The model under review builds one solid part; all positions refer to its coordinate system, in mm. A direction names the side the tool comes from. Give positions to 0.01 mm unless a question says otherwise; leave off trailing zeros. Order: outer loops, then holes, each group sorted by start corner. A loop starts at its lowest first (then second) coordinate and runs counter-clockwise, first axis right, second up.
```python
from build123d import *

# Parameters (mm, degrees)
SKETCH1_W                                       = 45
SKETCH1_H                                       = 50
BOSS_EXTRUDE1_DEPTH                             = 16
CUT_EXTRUDE1_DEPTH                              = 58.116109812
SKETCH4_W                                       = 24
SKETCH4_H                                       = 50
CUT_EXTRUDE2_DEPTH                              = 0.72
CUT_EXTRUDE3_DEPTH                              = 58.116109812
SKETCH8_R                                       = 7.5
CUT_EXTRUDE4_DEPTH                              = 0.72
CSK_FOR_M6_FLAT_HEAD_MACHINE_SCREW1_D           = 7
CSK_FOR_M6_FLAT_HEAD_MACHINE_SCREW1_CSINK_D     = 12.6
CSK_FOR_M6_FLAT_HEAD_MACHINE_SCREW1_CSINK_ANGLE = 90
CUT_EXTRUDE5_DEPTH                              = 2.5
FILLET1_R                                       = 1
FILLET2_R                                       = 1
FILLET4_R                                       = 0.5
CUT_EXTRUDE7_DEPTH                              = 11.5
SKETCH18_R                                      = 2.75
CUT_EXTRUDE8_DEPTH                              = 14.5
SKETCH19_R                                      = 2.75
CUT_EXTRUDE9_DEPTH                              = 10
SKETCH21_W                                      = 8.99
SKETCH21_H                                      = 50
BOSS_EXTRUDE2_DEPTH                             = 0.6
CHAMFER1_SIZE                                   = 4
FILLET5_R                                       = 1
CHAMFER2_SIZE                                   = 1


with BuildPart() as part:
    # Sketch1 → Boss-Extrude1 (new body)
    with BuildSketch(Plane(origin=(0, 0, 0), x_dir=(1, 0, 0), z_dir=(0, 1, 0))):
        Rectangle(SKETCH1_W, SKETCH1_H)
    extrude(amount=BOSS_EXTRUDE1_DEPTH)

    # Sketch3 → Cut-Extrude1 (cut, through all)
    with BuildSketch(Plane.XY.offset(25)):
        Polygon((-13.5, 16), (-17.5, 12), (22.5, 12), (22.5, 16), align=None)
    extrude(amount=-CUT_EXTRUDE1_DEPTH, mode=Mode.SUBTRACT)

    # Sketch4 → Cut-Extrude2 (cut)
    with BuildSketch(Plane(origin=(0, 12, 0), x_dir=(1, 0, 0), z_dir=(0, 1, 0))):
        with Locations((2.5, 0)):
            Rectangle(SKETCH4_W, SKETCH4_H)
    extrude(amount=-CUT_EXTRUDE2_DEPTH, mode=Mode.SUBTRACT)

    # Sketch5 → Cut-Extrude3 (cut, through all)
    with BuildSketch(Plane.XY.offset(25)):
        Polygon((-22.5, 16), (-13.5, 16), (-13.51, 15.99), (-22.5, 15.99), align=None)
    extrude(amount=-CUT_EXTRUDE3_DEPTH, mode=Mode.SUBTRACT)

    # Sketch8 → Cut-Extrude4 (cut)
    with BuildSketch(Plane(origin=(0, 11.28, 0), x_dir=(1, 0, 0), z_dir=(0, 1, 0))):
        with Locations(Location((2.5, 0, 0), (0, 0, 180))):
            Circle(SKETCH8_R)
    extrude(amount=-CUT_EXTRUDE4_DEPTH, mode=Mode.SUBTRACT)

    # CSK for M6 Flat Head Machine Screw1 (through all)
    with Locations(Plane(origin=(0, 10.56, 0), x_dir=(1, 0, 0), z_dir=(0, 1, 0))):
        with Locations((2.5, 0)):
            CounterSinkHole(CSK_FOR_M6_FLAT_HEAD_MACHINE_SCREW1_D / 2, CSK_FOR_M6_FLAT_HEAD_MACHINE_SCREW1_CSINK_D / 2, counter_sink_angle=CSK_FOR_M6_FLAT_HEAD_MACHINE_SCREW1_CSINK_ANGLE)

    # Sketch12 → Cut-Extrude5 (cut)
    with BuildSketch(Plane(origin=(0, 11.28, 0), x_dir=(1, 0, 0), z_dir=(0, 1, 0))):
        with BuildLine():
            Line((7.5, 16.6), (-2.5, 16.6))
            ThreePointArc((-2.5, 16.6), (-3.207106781, 16.892893219), (-3.5, 17.6))
            Line((-3.5, 17.6), (-3.5, 25))
            Line((-3.5, 25), (8.5, 25))
            Line((8.5, 25), (8.5, 17.6))
            ThreePointArc((8.5, 17.6), (8.207106781, 16.892893219), (7.5, 16.6))
        make_face()
    cut_extrude5 = extrude(amount=-CUT_EXTRUDE5_DEPTH, mode=Mode.SUBTRACT)

    # Fillet1
    fillet1_edges = [part.edges().sort_by_distance(p)[0] for p in [
        (-3.5, 10.03, -25),
        (8.5, 10.03, -25),
    ]]
    fillet(fillet1_edges, radius=FILLET1_R)

    # Mirror2: Cut-Extrude5 across plane
    add(cut_extrude5.mirror(Plane.XY), mode=Mode.SUBTRACT)

    # Fillet2
    # the kernel refuses this fillet: 1 mm, written as the material it takes off along each edge
    with BuildSketch(Plane(origin=(7.5, 11.28, 17.6), x_dir=(1, 0, 0), z_dir=(0, 0, 1))) as fillet2_piece_1:
        with BuildLine():
            CenterArc((1 + FILLET2_R, -FILLET2_R), FILLET2_R, 90, 90)
            Line((1, -FILLET2_R), (1 - FILLET2_R * 0.02, -FILLET2_R))
            Line((1 - FILLET2_R * 0.02, -FILLET2_R), (1 - FILLET2_R * 0.02, FILLET2_R * 0.02))
            Line((1 - FILLET2_R * 0.02, FILLET2_R * 0.02), (1 + FILLET2_R, FILLET2_R * 0.02))
            Line((1 + FILLET2_R, FILLET2_R * 0.02), (1 + FILLET2_R, 0))
        make_face()
    revolve(axis=Axis((7.5, 11.28, 17.6), (0, 1, 0)), revolution_arc=90, mode=Mode.SUBTRACT)
    with BuildSketch(Plane(origin=(8.5, 11.28, 27.5), x_dir=(1, 0, 0), z_dir=(0, 0, -1)), Plane(origin=(-3.5, 11.28, 17.6), x_dir=(-1, 0, 0), z_dir=(0, 0, 1))) as fillet2_piece_2:
        with BuildLine():
            CenterArc((FILLET2_R, FILLET2_R), FILLET2_R, 180, 90)
            Line((0, FILLET2_R), (-FILLET2_R * 0.02, FILLET2_R))
            Line((-FILLET2_R * 0.02, FILLET2_R), (-FILLET2_R * 0.02, -FILLET2_R * 0.02))
            Line((-FILLET2_R * 0.02, -FILLET2_R * 0.02), (FILLET2_R, -FILLET2_R * 0.02))
            Line((FILLET2_R, -FILLET2_R * 0.02), (FILLET2_R, 0))
        make_face()
    extrude(amount=9.9, mode=Mode.SUBTRACT)
    with BuildSketch(Plane(origin=(-2.5, 11.28, 17.6), x_dir=(0, 0, -1), z_dir=(1, 0, 0))) as fillet2_piece_3:
        with BuildLine():
            CenterArc((1 + FILLET2_R, -FILLET2_R), FILLET2_R, 90, 90)
            Line((1, -FILLET2_R), (1 - FILLET2_R * 0.02, -FILLET2_R))
            Line((1 - FILLET2_R * 0.02, -FILLET2_R), (1 - FILLET2_R * 0.02, FILLET2_R * 0.02))
            Line((1 - FILLET2_R * 0.02, FILLET2_R * 0.02), (1 + FILLET2_R, FILLET2_R * 0.02))
            Line((1 + FILLET2_R, FILLET2_R * 0.02), (1 + FILLET2_R, 0))
        make_face()
    revolve(axis=Axis((-2.5, 11.28, 17.6), (0, 1, 0)), revolution_arc=90, mode=Mode.SUBTRACT)
    with BuildSketch(Plane(origin=(7.5, 11.28, 16.6), x_dir=(0, 0, -1), z_dir=(-1, 0, 0))) as fillet2_piece_4:
        with BuildLine():
            CenterArc((FILLET2_R, FILLET2_R), FILLET2_R, 180, 90)
            Line((0, FILLET2_R), (-FILLET2_R * 0.02, FILLET2_R))
            Line((-FILLET2_R * 0.02, FILLET2_R), (-FILLET2_R * 0.02, -FILLET2_R * 0.02))
            Line((-FILLET2_R * 0.02, -FILLET2_R * 0.02), (FILLET2_R, -FILLET2_R * 0.02))
            Line((FILLET2_R, -FILLET2_R * 0.02), (FILLET2_R, 0))
        make_face()
    extrude(amount=10, mode=Mode.SUBTRACT)
    with BuildSketch(Plane(origin=(-4.5, 11.28, -25), x_dir=(0, 0, 1), z_dir=(-1, 0, 0)), Plane(origin=(14.5, 11.28, -25), x_dir=(0, 0, 1), z_dir=(-1, 0, 0))) as fillet2_piece_5:
        with BuildLine():
            CenterArc((FILLET2_R, -FILLET2_R), FILLET2_R, 90, 90)
            Line((0, -FILLET2_R), (-FILLET2_R * 0.02, -FILLET2_R))
            Line((-FILLET2_R * 0.02, -FILLET2_R), (-FILLET2_R * 0.02, FILLET2_R * 0.02))
            Line((-FILLET2_R * 0.02, FILLET2_R * 0.02), (FILLET2_R, FILLET2_R * 0.02))
            Line((FILLET2_R, FILLET2_R * 0.02), (FILLET2_R, 0))
        make_face()
    extrude(amount=5, mode=Mode.SUBTRACT)
    with BuildSketch(Plane(origin=(2.5, 11.28, 0), x_dir=(-1, 0, 0), z_dir=(0, 0, -1))) as fillet2_piece_6:
        with BuildLine():
            CenterArc((8.46, -1), FILLET2_R, 90, 73.739795292)
            Line((7.5, -0.72), (7.4808, -0.7144))
            ThreePointArc((7.4808, -0.7144), (7.48, -0.36), (7.48, 0))
            Line((7.48, 0), (7.5, 0.02))
            Line((7.5, 0.02), (8.46, 0.02))
            Line((8.46, 0.02), (8.46, 0))
        make_face()
    revolve(axis=Axis((2.5, 11.28, 0), (0, 1, 0)), mode=Mode.SUBTRACT)
    with BuildSketch(Plane(origin=(7.5, 11.28, -17.6), x_dir=(1, 0, 0), z_dir=(0, 0, -1))) as fillet2_piece_7:
        with BuildLine():
            CenterArc((1 + FILLET2_R, FILLET2_R), FILLET2_R, 180, 90)
            Line((1, FILLET2_R), (1 - FILLET2_R * 0.02, FILLET2_R))
            Line((1 - FILLET2_R * 0.02, FILLET2_R), (1 - FILLET2_R * 0.02, -FILLET2_R * 0.02))
            Line((1 - FILLET2_R * 0.02, -FILLET2_R * 0.02), (1 + FILLET2_R, -FILLET2_R * 0.02))
            Line((1 + FILLET2_R, -FILLET2_R * 0.02), (1 + FILLET2_R, 0))
        make_face()
    revolve(axis=Axis((7.5, 11.28, -17.6), (0, -1, 0)), revolution_arc=90, mode=Mode.SUBTRACT)
    with BuildSketch(Plane(origin=(8.5, 11.28, -24), x_dir=(1, 0, 0), z_dir=(0, 0, 1)), Plane(origin=(-3.5, 11.28, -17.6), x_dir=(-1, 0, 0), z_dir=(0, 0, -1))) as fillet2_piece_8:
        with BuildLine():
            CenterArc((FILLET2_R, -FILLET2_R), FILLET2_R, 90, 90)
            Line((0, -FILLET2_R), (-FILLET2_R * 0.02, -FILLET2_R))
            Line((-FILLET2_R * 0.02, -FILLET2_R), (-FILLET2_R * 0.02, FILLET2_R * 0.02))
            Line((-FILLET2_R * 0.02, FILLET2_R * 0.02), (FILLET2_R, FILLET2_R * 0.02))
            Line((FILLET2_R, FILLET2_R * 0.02), (FILLET2_R, 0))
        make_face()
    extrude(amount=6.4, mode=Mode.SUBTRACT)
    with BuildSketch(Plane(origin=(-2.5, 11.28, -17.6), x_dir=(0, 0, 1), z_dir=(1, 0, 0))) as fillet2_piece_9:
        with BuildLine():
            CenterArc((1 + FILLET2_R, FILLET2_R), FILLET2_R, 180, 90)
            Line((1, FILLET2_R), (1 - FILLET2_R * 0.02, FILLET2_R))
            Line((1 - FILLET2_R * 0.02, FILLET2_R), (1 - FILLET2_R * 0.02, -FILLET2_R * 0.02))
            Line((1 - FILLET2_R * 0.02, -FILLET2_R * 0.02), (1 + FILLET2_R, -FILLET2_R * 0.02))
            Line((1 + FILLET2_R, -FILLET2_R * 0.02), (1 + FILLET2_R, 0))
        make_face()
    revolve(axis=Axis((-2.5, 11.28, -17.6), (0, -1, 0)), revolution_arc=90, mode=Mode.SUBTRACT)
    with BuildSketch(Plane(origin=(7.5, 11.28, -16.6), x_dir=(0, 0, 1), z_dir=(-1, 0, 0))) as fillet2_piece_10:
        with BuildLine():
            CenterArc((FILLET2_R, -FILLET2_R), FILLET2_R, 90, 90)
            Line((0, -FILLET2_R), (-FILLET2_R * 0.02, -FILLET2_R))
            Line((-FILLET2_R * 0.02, -FILLET2_R), (-FILLET2_R * 0.02, FILLET2_R * 0.02))
            Line((-FILLET2_R * 0.02, FILLET2_R * 0.02), (FILLET2_R, FILLET2_R * 0.02))
            Line((FILLET2_R, FILLET2_R * 0.02), (FILLET2_R, 0))
        make_face()
    extrude(amount=10, mode=Mode.SUBTRACT)
    with BuildSketch(Plane(origin=(-4.5, 11.28, -24), x_dir=(0, 0, -1), z_dir=(-1, 0, 0))) as fillet2_piece_11:
        with BuildLine():
            CenterArc((1 - FILLET2_R, FILLET2_R), FILLET2_R, 270, 90)
            Line((1, FILLET2_R), (1 + FILLET2_R * 0.02, FILLET2_R))
            Line((1 + FILLET2_R * 0.02, FILLET2_R), (1 + FILLET2_R * 0.02, 0))
            Line((1 + FILLET2_R * 0.02, 0), (1, -FILLET2_R * 0.02))
            Line((1, -FILLET2_R * 0.02), (1 - FILLET2_R, -FILLET2_R * 0.02))
            Line((1 - FILLET2_R, -FILLET2_R * 0.02), (1 - FILLET2_R, 0))
        make_face()
    revolve(axis=Axis((-4.5, 11.28, -24), (0, -1, 0)), revolution_arc=90, mode=Mode.SUBTRACT)
    with BuildSketch(Plane(origin=(9.5, 11.28, -24), x_dir=(0, 0, -1), z_dir=(1, 0, 0))) as fillet2_piece_12:
        with BuildLine():
            CenterArc((1 - FILLET2_R, -FILLET2_R), FILLET2_R, 0, 90)
            Line((1, -FILLET2_R), (1 + FILLET2_R * 0.02, -FILLET2_R))
            Line((1 + FILLET2_R * 0.02, -FILLET2_R), (1 + FILLET2_R * 0.02, 0))
            Line((1 + FILLET2_R * 0.02, 0), (1, FILLET2_R * 0.02))
            Line((1, FILLET2_R * 0.02), (1 - FILLET2_R, FILLET2_R * 0.02))
            Line((1 - FILLET2_R, FILLET2_R * 0.02), (1 - FILLET2_R, 0))
        make_face()
    revolve(axis=Axis((9.5, 11.28, -24), (0, 1, 0)), revolution_arc=90, mode=Mode.SUBTRACT)

    # Fillet4
    fillet4_edges = [part.edges().sort_by_distance(p)[0] for p in [
        (-17.5, 12, 0),
    ]]
    fillet(fillet4_edges, radius=FILLET4_R)

    # Sketch14 → Cut-Extrude7 (cut)
    with BuildSketch(Plane(origin=(0, 12, 0), x_dir=(1, 0, 0), z_dir=(0, 1, 0))):
        Polygon((19.5, -8), (17.5, -8), (17.5, -3.45), (16.1, -3.45), (16.1, 3.45), (17.5, 3.45), (17.5, 8), (19.5, 8), align=None)
    extrude(amount=-CUT_EXTRUDE7_DEPTH, mode=Mode.SUBTRACT)

    # Sketch18 → Cut-Extrude8 (cut)
    with BuildSketch(Plane(origin=(22.5, 0, 0), x_dir=(0, 0, -1), z_dir=(1, 0, 0))):
        with Locations((0, 6)):
            Circle(SKETCH18_R)
    extrude(amount=-CUT_EXTRUDE8_DEPTH, mode=Mode.SUBTRACT)

    # Sketch19 → Cut-Extrude9 (cut)
    with BuildSketch(Plane(origin=(22.5, 0, 0), x_dir=(0, 0, -1), z_dir=(1, 0, 0))):
        with Locations((-16, 6)):
            Circle(SKETCH19_R)
        with Locations((16, 6)):
            Circle(SKETCH19_R)
    extrude(amount=-CUT_EXTRUDE9_DEPTH, mode=Mode.SUBTRACT)

    # Sketch21 → Boss-Extrude2 (add)
    with BuildSketch(Plane(origin=(0, 15.99, 0), x_dir=(1, 0, 0), z_dir=(0, 1, 0))):
        with Locations((-18.005, 0)):
            Rectangle(SKETCH21_W, SKETCH21_H)
    extrude(amount=BOSS_EXTRUDE2_DEPTH)

    # Chamfer1
    chamfer1_edges = [part.edges().sort_by_distance(p)[0] for p in [
        (-22.5, 8.295, 25),
        (-22.5, 8.295, -25),
    ]]
    chamfer(chamfer1_edges, length=CHAMFER1_SIZE)

    # Fillet5
    fillet5_edges = [part.edges().sort_by_distance(p)[0] for p in [
        (-22.5, 16.59, 0),
    ]]
    fillet(fillet5_edges, radius=FILLET5_R)

    # Chamfer2
    chamfer2_edges = [part.edges().sort_by_distance(p)[0] for p in [
        (18.5, 12, 8),
        (18.5, 12, -8),
    ]]
    chamfer(chamfer2_edges, length=CHAMFER2_SIZE)


solid = part.part
```
Item 1: Clearance check with flat-ended pins moving along their axes: pin 1 Ø1.5 at (x, z) = (-8.5, -20) entering from +Y; pin 2 Ø0.5 at (y, z) = (16.5, -5.5) entering from +X; pin 3 Ø1 at (y, z) = (6.5, -18) entering from +X. State where each tip first meets the part, or that it passes through.
Values found:
pin 1: stops at y = 11.28
pin 2: stops at x = -13.51
pin 3: stops at x = 12.5
Item 2: Take a section at C-C (y = 2.5). Give the boundary of the cut face in (x, z).
Values found:
outline: (-22.5, -21) - (-18.5, -25) - (22.5, -25) - (22.5, 25) - (-18.5, 25) - (-22.5, 21) - close; hole circle Ø7 at (2.5, 0); hole (16.1, -3.45) - (17.5, -3.45) - (17.5, -8) - (19.5, -8) - (19.5, 8) - (17.5, 8) - (17.5, 3.45) - (16.1, 3.45) - close
Item 3: For faces 1 (the flat face through (3, 8.78, 21)), 2 (the flat face through (17.5, 6, 6)), 3 (the flat face through (3, 8.78, -21)), list the 3-axis set-ups (+Z, -Z, +X, -X, +Y, -Y) from which the entire face can be reached by the end or side of a thin tool; tool diameter is ignored.
Values found:
face 1: +Z, +Y
face 2: +Y
face 3: -Z, +Y
Item 4: Draft analysis for pull direction Y (two halves, no side actions). For faces 4 (the cylindrical face through (17.57, 4.327, 18.182)), 5 (the conical face through (-0.968, 7.896, -1.092)), 6 (the flat face through (-3.5, 10, -21)), state which applies: released by +Y, released by -Y, zero draft, split by the parting line, or undercut.
Values found:
face 4: undercut
face 5: released by +Y
face 6: zero draft
Item 5: Take a section at A-A (x = 2.5). Give the boundary of the cut face in (y, z), and give its area (3 significant figures).
Values found:
outline: (0, -25) - (8.78, -25) - (8.78, -16.6) - (10.28, -16.6) arc R1 ccw to (11.28, -15.6) - (11.28, -8.46) arc R1 ccw to (10.56, -7.5) - (10.56, -6.3) - (7.76, -3.5) - (0, -3.5) - close; (0, 3.5) - (7.76, 3.5) - (10.56, 6.3) - (10.56, 7.5) arc R1 ccw to (11.28, 8.46) - (11.28, 15.6) arc R1 ccw to (10.28, 16.6) - (8.78, 16.6) - (8.78, 25) - (0, 25) - close
area: 429 mm2
Item 6: For line 1 (Y direction, x = 21.85, z = 0); line 2 (Y direction, x = 12.75, z = 0); line 3 (Z direction, x = 2.5, y = 1.5), list the stretches that pass through material, from the lowest coordinate up.
Values found:
line 1: y = 0 to 3.25, 8.75 to 12
line 2: y = 0 to 3.25, 8.75 to 11.28
line 3: z = -25 to -3.5, 3.5 to 25
Item 7: Take a section at D-D (z = 12). Give the boundary of the cut face in (x, y).
Values found:
outline: (-22.5, 0) - (22.5, 0) - (22.5, 12) - (14.5, 12) - (14.5, 11.28) - (-9.5, 11.28) - (-9.5, 12) - (-16.29, 12) arc R0.5 cw to (-16.65, 12.85) - (-13.51, 15.99) - (-13.51, 16.59) - (-21.5, 16.59) arc R1 ccw to (-22.5, 15.59) - close
